from build123d import *

# Parameters (mm, degrees)
F0_W = 8.2200646866
F0_H = 9.3895217869


# Not quite as in the source:
# - a feature names something its author has since deleted; it is built from what else it names


with BuildPart() as f1:
    # F0 (on Front) → F1 (revolve)
    with BuildSketch(Plane.XZ):
        with BuildLine():
            Line((0, 19), (0, 0))
            Line((0, 0), (0.6, 0))
            Line((0.6, 0), (0.6, 3.5557271383))
            Line((0.6, 3.5557271383), (11.9, 3.5557271383))
            Line((11.9, 3.5557271383), (11.9, 16.2557271383))
            Line((11.9, 16.2557271383), (3.2369840445, 16.2557271383))
            ThreePointArc((3.2369840445, 16.2557271383), (5.2521158412, 17.0766330758), (6.1823196963, 19.0437028519))
            Line((6.1823196963, 19.0437028519), (6.3827879741, 19.0437028519))
            ThreePointArc((6.3827879741, 19.0437028519), (3.1678853473, 22.4552809766), (0, 19))
        make_face()
        with Locations((6.2782712048, 9.8272700561)):
            Rectangle(F0_W, F0_H, mode=Mode.SUBTRACT)
    revolve(axis=Axis((139.7, 0, -5.7849194854), (0, 0, -1)))


solid = f1.part
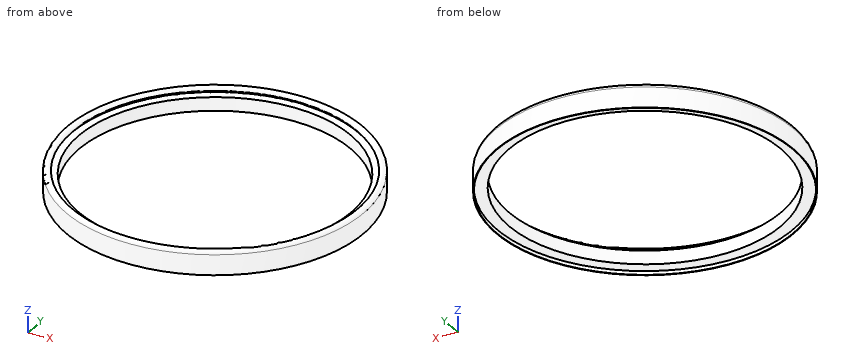
The model under review builds one solid part; all positions refer to its coordinate system, in mm. Give positions to 0.01 mm unless a question says otherwise; leave off trailing zeros. Order: outer loops, then holes, each group sorted by start corner. A loop starts at its lowest first (then second) coordinate and runs counter-clockwise, first axis right, second up. Notation, with made-up numbers: M 20,15.25 L 58,15.25 A17 ccw 58,25.25 Z; hole C -39,-13.75 d11. An arc over 180 degrees is marked long. One line per question, with ' | ' between items. Start each with the question number.
1) Consider section C-C, the plane x = 139.7. Give the boundary of the cut face in (y, z), then the cut area to 3 significant figures.
2) Consider section A-A, the plane z = 11. Give the boundary of the cut face in (x, y).
3) Clearance check with flat-ended pins moving along their axes: P1, Ø1.5, axis at x = 135, z = 15.5, coming from the -Y side; P2, Ø12, axis at y = 63.5, z = 7, coming from the +X side; P3, Ø6, axis at y = -81, z = 7.5, coming from the -X side. State where each tip first meets the part, or that it passes through.
4) Wall thickness on L1, parallel to Y at x = 139.7, z = 10.5; L2, parallel to X at y = 61, z = 12.5; L3, parallel to Y at x = 257, z = 8.5: over which ranges is each line inside the solid? List them lowest first. Write a range as from..to.
5) Consider section B-B, the plane y = 0. Give the boundary of the cut face in (x, z).
Found:
1) outline: M -139.7,0 L -139.1,0 L -139.1,3.56 L -127.8,3.56 L -127.8,16.26 L -136.46,16.26 A3 ccw -133.52,19.04 L -133.32,19.04 A3.2 ccw long -139.7,19 Z; M 127.8,3.56 L 139.1,3.56 L 139.1,0 L 139.7,0 L 139.7,19 A3.2 ccw long 133.32,19.04 L 133.52,19.04 A3 ccw 136.46,16.26 L 127.8,16.26 Z; hole M -137.53,5.13 L -129.31,5.13 L -129.31,14.52 L -137.53,14.52 Z; hole M 129.31,5.13 L 137.53,5.13 L 137.53,14.52 L 129.31,14.52 Z | area: 218 mm²
2) outline: C 139.7,0 d279.4; C 139.7,0 d258.62; hole C 139.7,0 d275.06; hole C 139.7,0 d255.6
3) P1: stops at y = -139.64 | P2: stops at x = 267.02 | P3: stops at x = 23.8
4) L1: y = -139.7..-137.53, -129.31..-127.8, 127.8..129.31, 137.53..139.7 | L2: x = 14.02..16.44, 25.68..27.4, 252..253.72, 262.96..265.38 | L3: y = -75.87..-71.8, -54.43..-50.73, 50.73..54.43, 71.8..75.87
5) outline: M 0,0 L 0.6,0 L 0.6,3.56 L 11.9,3.56 L 11.9,16.26 L 3.24,16.26 A3 ccw 6.18,19.04 L 6.38,19.04 A3.2 ccw long 0,19 Z; M 267.5,3.56 L 278.8,3.56 L 278.8,0 L 279.4,0 L 279.4,19 A3.2 ccw long 273.02,19.04 L 273.22,19.04 A3 ccw 276.16,16.26 L 267.5,16.26 Z; hole M 2.17,5.13 L 10.39,5.13 L 10.39,14.52 L 2.17,14.52 Z; hole M 269.01,5.13 L 277.23,5.13 L 277.23,14.52 L 269.01,14.52 Z
